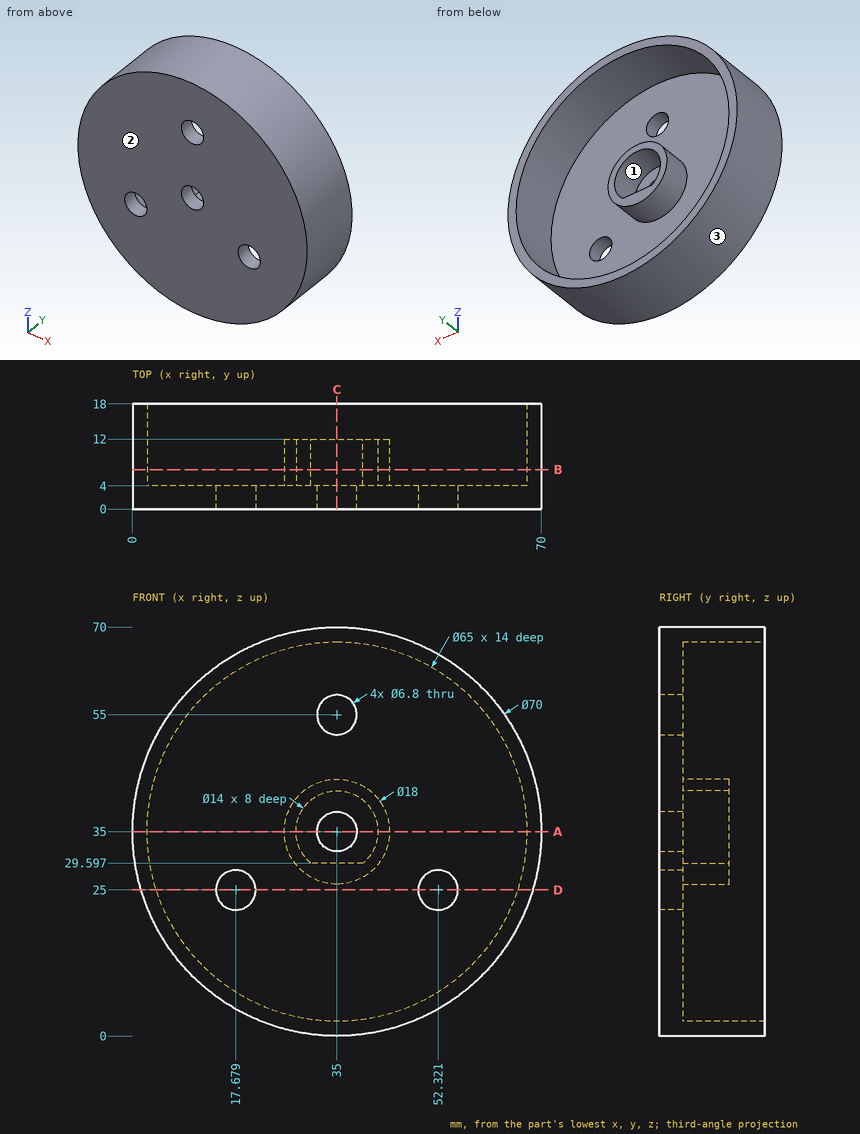
Part print with two shaded views. Sizes in mm from the minimum x, y, z corner. Round coordinates to 2 decimals unless told otherwise and drop trailing zeros. Loops run counter-clockwise (first coordinate to the right, second up) from the corner with the lowest first, then second, coordinate; pieces in that order, holes last. Notation, with made-up numbers: M 44,36.25 L 83,36.25 A21 cw 83,57.25 Z; hole C 6,16.5 d7. An arc over 180 degrees is marked long. Put each result on its own line as item: value. Start each with the question number.
Item 1: Drill centre lines: line 1 along X through (y, z) = (5.75, 35); line 2 along X through (y, z) = (4.75, 30.5) (1 decimal); line 3 along X through (y, z) = (2.4, 25). Where is each one in solid material? Low to high.
Item 2: Drop flat-ended pins along their axis: P1, Ø8, axis at y = 8.5, z = 23.5, coming from the -X side; P2, Ø1, axis at x = 26.5, y = 14.5, coming from the +Z side; P3, Ø6, axis at x = 45, z = 55, coming from the +Y side; P4, Ø5.5, axis at x = 35, z = 55, coming from the +Y side. Give the stop position or say it passes through.
Item 3: Cut at D-D (z = 25). List the corners of the cut face in (x, y).
Item 4: Cut at B-B (y = 6.75). List the corners of the cut face in (x, z).
Item 5: Cut at C-C (x = 35). List the corners of the cut face in (y, z).
Item 6: Mould opens along X. For the marked faces 1, 2 and 3 say: released by +X, released by -X, zero draft, split by the parting line, or undercut.
Item 7: Cut at A-A (z = 35). List the corners of the cut face in (x, y).
Answer block:
1. line 1: 0 to 2.5, 26 to 28, 42 to 44, 67.5 to 70
1. line 2: 0.3 to 2.8, 27.2 to 29.6, 40.4 to 42.8, 67.2 to 69.7
1. line 3: 1.46 to 14.28, 21.08 to 48.92, 55.72 to 68.54
2. P1: x = 0.81
2. P2: z = 69.07
2. P3: y = 4
2. P4: through
3. outline: M 1.46,0 L 14.28,0 L 14.28,4 L 4.08,4 L 4.08,18 L 1.46,18 Z; M 21.08,0 L 48.92,0 L 48.92,4 L 21.08,4 Z; M 55.72,0 L 68.54,0 L 68.54,18 L 65.92,18 L 65.92,4 L 55.72,4 Z
4. outline: C 35,35 d70; C 35,35 d18; hole C 35,35 d65; hole M 30.55,29.6 L 39.45,29.6 A7 ccw long Z
5. outline: M 0,0 L 18,0 L 18,2.5 L 4,2.5 L 4,26 L 12,26 L 12,29.6 L 4,29.6 L 4,31.6 L 0,31.6 Z; M 0,38.4 L 4,38.4 L 4,42 L 12,42 L 12,44 L 4,44 L 4,51.6 L 0,51.6 Z; M 0,58.4 L 4,58.4 L 4,67.5 L 18,67.5 L 18,70 L 0,70 Z
6. face 1: undercut
6. face 2: zero draft
6. face 3: split by the parting line
7. outline: M 0,0 L 31.6,0 L 31.6,4 L 28,4 L 28,12 L 26,12 L 26,4 L 2.5,4 L 2.5,18 L 0,18 Z; M 38.4,0 L 70,0 L 70,18 L 67.5,18 L 67.5,4 L 44,4 L 44,12 L 42,12 L 42,4 L 38.4,4 Z
